Job drawing, mm, ordinate dimensions from the low corner. One solid piece. Coordinates: 2 decimals unless noted, no trailing zeros. Order: outer loops, then holes, each group sorted by start corner. A loop starts at its lowest first (then second) coordinate and runs counter-clockwise, first axis right, second up. Notation, with made-up numbers: (-3, -26.75) - (15, -26.75) arc R18 ccw to (15, -14.75) - close; hole circle Ø10 at (29, 3.5). An arc over 180 degrees is marked (long way). Use a Markdown table: item, result. Add a question column.
1) Drop flat-ended pins along their axis: P1, Ø1.8, axis at x = 25.5, y = 68.5, coming from the -Z side; P2, Ø1.5, axis at y = 2, z = 9, coming from the -X side; P3, Ø2.5, axis at y = 77.1, z = 14, coming from the +X side. Give the stop position or say it passes through.
2) Saw through at B-B on z = 10. List the corners of the cut face in (x, y).
3) Saw through at A-A on x = 39.5. List the corners of the cut face in (y, z), then the cut area to 3 significant figures.
4) Two-plate mould, pull along Z, no slides. Class the marked faces 1, 2 and 3: +Z half, -Z half, draft (parallel to the pull), parting line (faces both ways), or undercut.
5) Wall check: L1, parallel to Y at x = 25.5, z = 2.9; L2, parallel to X at y = 68.5, z = 1.9; L3, parallel to Z at x = 48.9, y = 77.1. Give the ranges that are in metal, low to high. Write a range as [from, to].
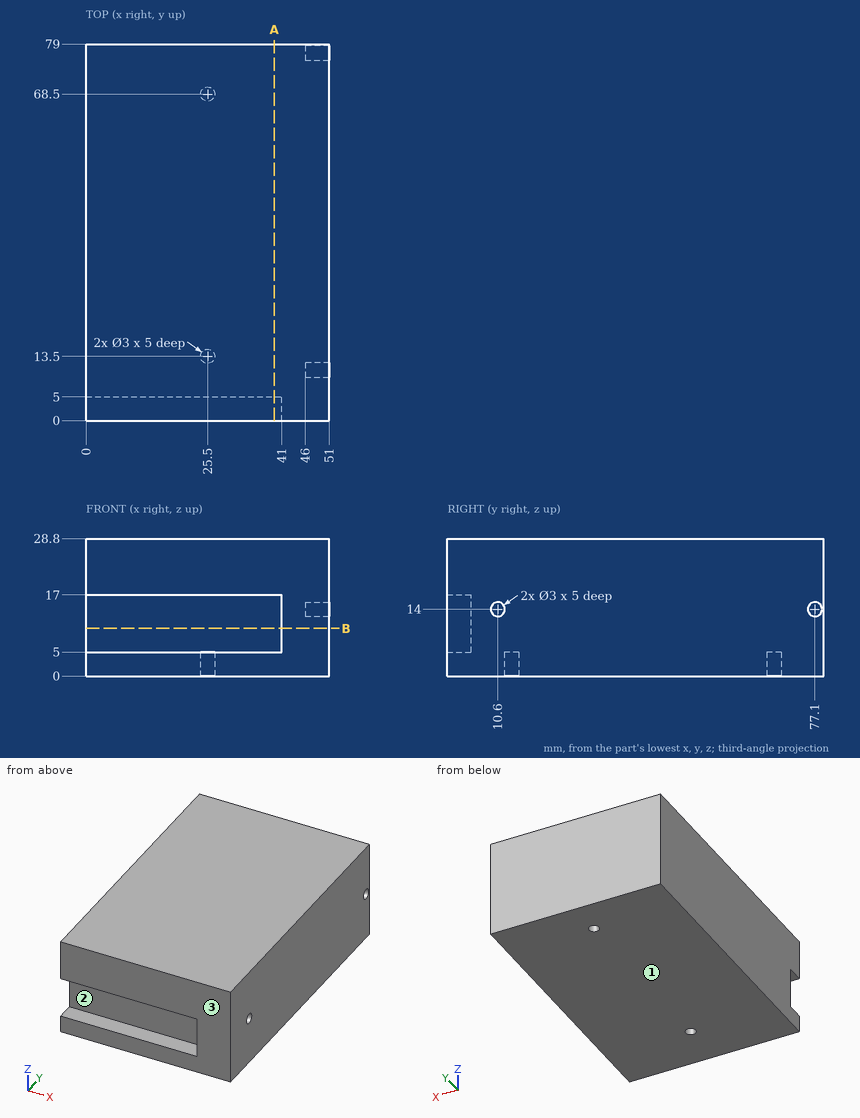
Results are:
| question | item | result |
|---|---|---|
| 1 | P1 | z = 5 |
| 1 | P2 | x = 41 |
| 1 | P3 | x = 46 |
| 2 | outline | (0, 5) - (41, 5) - (41, 0) - (51, 0) - (51, 79) - (0, 79) - close |
| 3 | outline | (0, 0) - (79, 0) - (79, 28.8) - (0, 28.8) - (0, 17) - (5, 17) - (5, 5) - (0, 5) - close |
| 3 | area | 2,220 mm2 |
| 4 | face 1 | -Z half |
| 4 | face 2 | undercut |
| 4 | face 3 | draft |
| 5 | L1 | [0, 12], [15, 67], [70, 79] |
| 5 | L2 | [0, 24], [27, 51] |
| 5 | L3 | [0, 12.5], [15.5, 28.8] |
